from build123d import *

# Parameters (mm, degrees)
BOSS_EXTRUDE1_DEPTH = 10
CUT_EXTRUDE1_DEPTH  = 3
SKETCH3_R           = 1.65
CUT_EXTRUDE2_DEPTH  = 6


with BuildPart() as part:
    # Sketch1 → Boss-Extrude1 (new body)
    with BuildSketch(Plane.XY):
        with BuildLine():
            Line((0, 1), (0, 5))
            ThreePointArc((0, 5), (0.292893219, 5.707106781), (1, 6))
            Line((1, 6), (9, 6))
            ThreePointArc((9, 6), (9.707106781, 5.707106781), (10, 5))
            Line((10, 5), (10, 3))
            ThreePointArc((10, 3), (10.292893219, 2.292893219), (11, 2))
            Line((11, 2), (18, 2))
            ThreePointArc((18, 2), (23.543277195, 10.296100594), (13.757359313, 12.242640687))
            ThreePointArc((13.757359313, 12.242640687), (12.459665918, 11.375549682), (10.928932188, 11.071067812))
            ThreePointArc((10.928932188, 11.071067812), (9.928932188, 12.071067812), (10.928932188, 13.071067812))
            ThreePointArc((10.928932188, 13.071067812), (11.694299053, 13.223308747), (12.343145751, 13.656854249))
            ThreePointArc((12.343145751, 13.656854249), (25.39103626, 11.061467459), (18, 0))
            Line((18, 0), (1, 0))
            ThreePointArc((1, 0), (0.292893219, 0.292893219), (0, 1))
        make_face()
    extrude(amount=BOSS_EXTRUDE1_DEPTH)

    # Sketch2 → Cut-Extrude1 (cut)
    with BuildSketch(Plane(origin=(0, 6, 0), x_dir=(1, 0, 0), z_dir=(0, 1, 0))):
        Polygon((5, -1.651368439), (2.1, -3.325684219), (2.1, -6.674315781), (5, -8.348631561), (7.9, -6.674315781), (7.9, -3.325684219), align=None)
    extrude(amount=-CUT_EXTRUDE1_DEPTH, mode=Mode.SUBTRACT)

    # Sketch3 → Cut-Extrude2 (cut)
    with BuildSketch(Plane(origin=(0, 6, 0), x_dir=(1, 0, 0), z_dir=(0, 1, 0))):
        with Locations(Location((5, -5, 0), (0, 0, 270))):
            Circle(SKETCH3_R)
    extrude(amount=-CUT_EXTRUDE2_DEPTH, mode=Mode.SUBTRACT)


solid = part.part
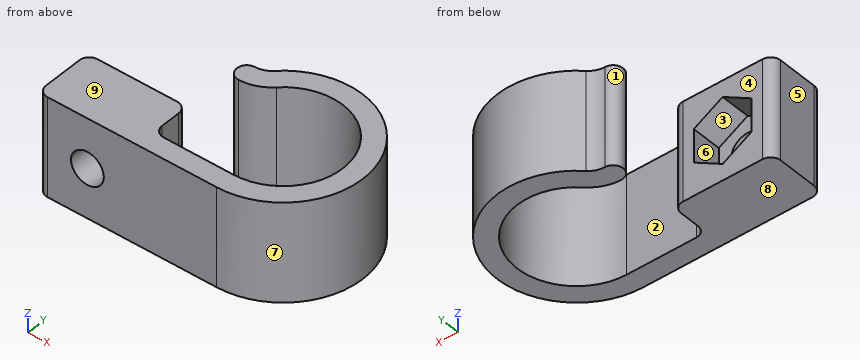
The model under review builds one solid part; all positions refer to its coordinate system, in mm. Face numbers are marked on the shaded views. A direction names the side the tool comes from. Round coordinates to 2 decimals unless told otherwise and drop trailing zeros. Loops run counter-clockwise (first coordinate to the right, second up) from the corner with the lowest first, then second, coordinate; pieces in that order, holes last. Notation, with made-up numbers: M 80.5,26.5 L 89.5,26.5 A19 ccw 89.5,30.5 Z; hole C -17,-26 d3. An arc over 180 degrees is marked long. Answer as a JSON object with one key per item and string values.
Item 1: We need section B-B, the plane x = 10.5. State the section outline as (y, z) points, and give its area (3 significant figures).
Check sheet entries:
{"outline": "M 0,0 L 2.13,0 L 2.13,10 L 0,10 Z; M 11.17,0 L 12.97,0 L 12.97,10 L 11.17,10 Z", "area": "39.4 mm2"}
Item 2: We need section D-D, the plane y = 8. State the section outline as (x, z) points, and give its area (3 significant figures).
Check sheet entries:
{"outline": "M 24,0 L 26,0 L 26,10 L 24,10 Z", "area": "20.0 mm2"}
Item 3: For line 1 along Y through (x, z) = (18, 6.75); line 2 along X through (y, z) = (13.25, 1.75); line 3 along Y through (x, z) = (5, 3.25), list the stretches that pass through material, from the lowest coordinate up.
Check sheet entries:
{"line 1": "0 to 2, 14 to 16", "line 2": "11.76 to 15.1, 20.9 to 24.04", "line 3": "0 to 3"}
Item 4: We need section A-A, the plane z = 5. State the section outline as (x, y) points.
Check sheet entries:
{"outline": "M 0,1 A1 ccw 1,0 L 3.35,0 L 3.35,3 L 2.1,3 L 2.1,6 L 1,6 A1 ccw 0,5 Z; M 6.65,0 L 18,0 A8 ccw long 12.34,13.66 A2 cw 10.93,13.07 A1 ccw 10.93,11.07 A4 ccw 13.76,12.24 A6 cw long 18,2 L 11,2 A1 cw 10,3 L 10,5 A1 ccw 9,6 L 7.9,6 L 7.9,3 L 6.65,3 Z"}
Item 5: Tool access review of the marked faces 1, 2, 3, 4 and 5: name each direction out of +Z, -Z, +X, -X, +Y, -Y from which nothing blocks a thin tool from reaching the whole face with its end or side.
Check sheet entries:
{"face 1": "+Z, -Z, -X", "face 2": "+Z, -Z", "face 3": "+Y", "face 4": "+Z, -Z, -X, +Y", "face 5": "+Z, -Z, -X, +Y, -Y"}
Item 6: We need section C-C, the plane z = 9. State the section outline as (x, y) points, and give its area (3 significant figures).
Check sheet entries:
{"outline": "M 0,1 A1 ccw 1,0 L 18,0 A8 ccw long 12.34,13.66 A2 cw 10.93,13.07 A1 ccw 10.93,11.07 A4 ccw 13.76,12.24 A6 cw long 18,2 L 11,2 A1 cw 10,3 L 10,5 A1 ccw 9,6 L 1,6 A1 ccw 0,5 Z", "area": "137 mm2"}
Item 7: Clearance check with flat-ended pins moving along their axes: P1, Ø1, axis at x = 23, z = 4, coming from the +Y side; P2, Ø2, axis at y = 12.5, z = 1.5, coming from the +X side; P3, Ø6, axis at y = 10.5, z = 4.5, coming from the -X side. State where each tip first meets the part, or that it passes through.
Check sheet entries:
{"P1": "y = 14.61", "P2": "x = 25.19", "P3": "x = 9.93"}
Item 8: The part is to be moulded in two halves that separate along Z. For the marked faces 6, 7, 8 and 9, say which applies: +Z half, -Z half, draft (parallel to the pull), parting line (faces both ways), or undercut.
Check sheet entries:
{"face 6": "undercut", "face 7": "draft", "face 8": "-Z half", "face 9": "+Z half"}
